Part print with two shaded views. Sizes in mm from the minimum x, y, z corner. Give positions to 0.01 mm unless a question says otherwise; leave off trailing zeros. Order: outer loops, then holes, each group sorted by start corner. A loop starts at its lowest first (then second) coordinate and runs counter-clockwise, first axis right, second up. Notation, with made-up numbers: M 13,-21.75 L 25,-21.75 A19 ccw 25,-14.75 Z; hole C 72,36.25 d3. An arc over 180 degrees is marked long. Write each question's results on one line, items separated by ' | '. Start each with the question number.
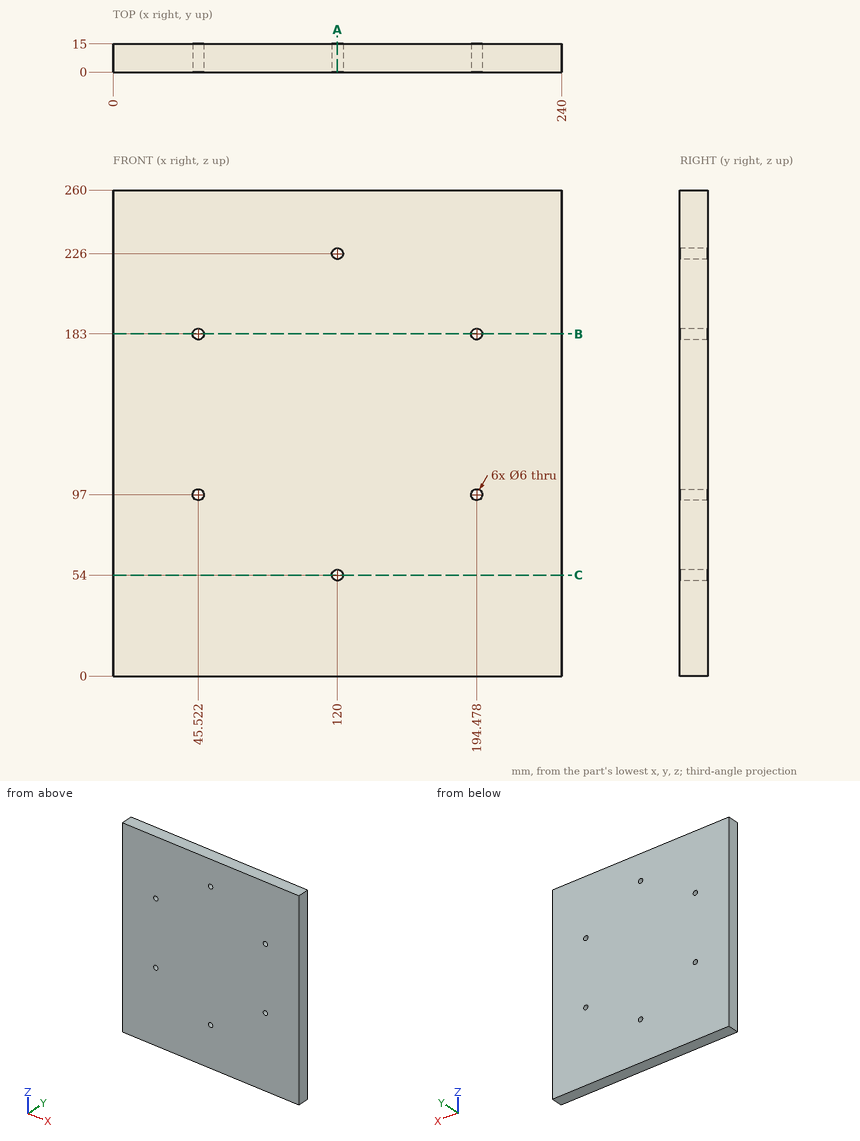
(1) Probe L1, parallel to X at y = 8.5, z = 183; L2, parallel to X at y = 9, z = 226; L3, parallel to X at y = 3, z = 55.5. List the from-to ranges inside material, lowest first.
(2) Drop a flat-ended pin along its axis: P1, Ø5, axis at x = 120, z = 54, coming from the -Y side. Give the stop position or say it passes through.
(3) Saw through at A-A on x = 120. Give the cut face in (y, z), plus the area to 3 significant figures.
(4) Saw through at B-B on z = 183. Give the cut face in (x, y), plus the area to 3 significant figures.
(5) Saw through at C-C on z = 54. Give the cut face in (x, y), plus the area to 3 significant figures.
Taken from the geometry:
1) L1: x = 0 to 42.52, 48.52 to 191.48, 197.48 to 240 | L2: x = 0 to 117, 123 to 240 | L3: x = 0 to 117.4, 122.6 to 240
2) P1: passes through
3) outline: M 0,0 L 15,0 L 15,51 L 0,51 Z; M 0,57 L 15,57 L 15,223 L 0,223 Z; M 0,229 L 15,229 L 15,260 L 0,260 Z | area: 3,720 mm²
4) outline: M 0,0 L 42.52,0 L 42.52,15 L 0,15 Z; M 48.52,0 L 191.48,0 L 191.48,15 L 48.52,15 Z; M 197.48,0 L 240,0 L 240,15 L 197.48,15 Z | area: 3,420 mm²
5) outline: M 0,0 L 117,0 L 117,15 L 0,15 Z; M 123,0 L 240,0 L 240,15 L 123,15 Z | area: 3,510 mm²
